Model file for the job. Use its own axes, mm. A direction names the side the tool comes from. Give positions to 0.01 mm unless a question says otherwise; leave off trailing zeros. Loops run counter-clockwise (first coordinate to the right, second up) from the corner with the lowest first, then second, coordinate; pieces in that order, holes last. Notation, with made-up numbers: M -22.5,-6.5 L 16.5,-6.5 A28 ccw 16.5,24.5 Z; hole C 88,47 d10. An arc over 180 degrees is marked long. Answer in a Markdown table with one row per item.
```python
from build123d import *

# Parameters (mm, degrees)
SKETCH1_W           = 34
SKETCH1_H           = 20
BOSS_EXTRUDE1_DEPTH = 1.1
SKETCH3_W           = 34
SKETCH3_H           = 18
BOSS_EXTRUDE2_DEPTH = 1.2
SKETCH4_W           = 5
SKETCH4_H           = 2.3
BOSS_EXTRUDE3_DEPTH = 0.5
SKETCH5_W           = 17
SKETCH5_H           = 2
BOSS_EXTRUDE4_DEPTH = 0.5
SKETCH6_W           = 17
SKETCH6_H           = 0.5
BOSS_EXTRUDE5_DEPTH = 20


with BuildPart() as part:
    # Sketch1 → Boss-Extrude1 (new body)
    with BuildSketch(Plane(origin=(0, 0, 0), x_dir=(1, 0, 0), z_dir=(0, 1, 0))):
        Rectangle(SKETCH1_W, SKETCH1_H)
    extrude(amount=BOSS_EXTRUDE1_DEPTH)

    # Sketch3 → Boss-Extrude2 (add)
    with BuildSketch(Plane(origin=(0, 1.1, 0), x_dir=(1, 0, 0), z_dir=(0, 1, 0))):
        with Locations((0, 1)):
            Rectangle(SKETCH3_W, SKETCH3_H)
    extrude(amount=BOSS_EXTRUDE2_DEPTH)

    # Sketch4 → Boss-Extrude3 (add)
    with BuildSketch(Plane.ZY.offset(17)):
        with Locations((-1, 1.15)):
            Rectangle(SKETCH4_W, SKETCH4_H)
    extrude(amount=BOSS_EXTRUDE3_DEPTH)

    # Sketch5 → Boss-Extrude4 (add)
    with BuildSketch(Plane(origin=(0, 1.1, 0), x_dir=(1, 0, 0), z_dir=(0, 1, 0))):
        with Locations((0, -9)):
            Rectangle(SKETCH5_W, SKETCH5_H)
    extrude(amount=BOSS_EXTRUDE4_DEPTH)

    # Sketch6 → Boss-Extrude5 (add)
    with BuildSketch(Plane(origin=(0, 1.6, 0), x_dir=(1, 0, 0), z_dir=(0, 1, 0))):
        with Locations((0, -10.25)):
            Rectangle(SKETCH6_W, SKETCH6_H)
    extrude(amount=-BOSS_EXTRUDE5_DEPTH)


solid = part.part
```
(1) Saw through at B-B, the plane z = -2.75. Give the cut face in (x, y), and give its area (4 significant figures).
Established:
| item | result |
|---|---|
| outline | M -17.5,0 L 17,0 L 17,2.3 L -17.5,2.3 Z |
| area | 79.35 mm2 |
(2) Which spindle directions (+Z, -Z, +X, -X, +Y, -Y) get a long thin tool onto all of the face, cutting with end or side? Do faces 1 (the flat face through (0, -9, 10)), 2 (the flat face through (-17, 1, 6)), 3 (the flat face through (-17, 1, -7)), 4 (the flat face through (13, 1.1, 9)), 5 (the flat face through (0, 1.6, 9)). Say none if no direction does.
Established:
| item | result |
|---|---|
| face 1 | -Z, +X, -X, -Y |
| face 2 | +Z, -X, +Y, -Y |
| face 3 | -Z, -X, +Y, -Y |
| face 4 | +Z, +X, +Y |
| face 5 | +Z, +X, -X, +Y |
(3) Saw through at A-A, the plane x = 4. Give the cut face in (y, z), and give its area (3 significant figures).
Established:
| item | result |
|---|---|
| outline | M -18.4,10 L 0,10 L 0,-10 L 2.3,-10 L 2.3,8 L 1.6,8 L 1.6,10.5 L -18.4,10.5 Z |
| area | 54.6 mm2 |
(4) Flat gauge pins, fed straight in: P1, Ø1, axis at x = -10, z = 7.5, coming from the -Y side; P2, Ø8.5, axis at x = -1.5, y = -7.5, coming from the -Z side; P3, Ø3, axis at y = -4.5, z = 9.5, coming from the +X side. Where does each tip first touch, or does it go through?
Established:
| item | result |
|---|---|
| P1 | stops at y = 0 |
| P2 | stops at z = 10 |
| P3 | stops at x = 8.5 |
(5) Saw through at C-C, the plane y = -9. Give the cut face in (x, z), and give its area (3 significant figures).
Established:
| item | result |
|---|---|
| outline | M -8.5,10 L 8.5,10 L 8.5,10.5 L -8.5,10.5 Z |
| area | 8.50 mm2 |
(6) Wall check: L1, parallel to Y at x = -6.5, z = 3; L2, parallel to Z at x = -6, y = -3; L3, parallel to Y at x = 1.5, z = 8.75. Give the ranges that are in metal, low to high.
Established:
| item | result |
|---|---|
| L1 | y = 0 to 2.3 |
| L2 | z = 10 to 10.5 |
| L3 | y = 0 to 1.6 |
(7) Saw through at D-D, the plane x = 13.5. Give the cut face in (y, z), and give its area (3 significant figures).
Established:
| item | result |
|---|---|
| outline | M 0,-10 L 2.3,-10 L 2.3,8 L 1.1,8 L 1.1,10 L 0,10 Z |
| area | 43.6 mm2 |
